The listing builds one solid part. Answer for the finished solid, in the listing's coordinates (mm). Face numbers are marked on the shaded views. Give positions to 0.01 mm unless a question says otherwise; leave off trailing zeros. Loops run counter-clockwise (first coordinate to the right, second up) from the corner with the lowest first, then second, coordinate; pieces in that order, holes last.
Item 1: Section B-B, the plane x = 0 is taken. Give the vertices of the cut face in (y, z).
Item 2: Each of these flat-tipped pins is pushed along its axis until it touches: pin 1 Ø5 at (x, z) = (-7, 7) entering from +Y; pin 2 Ø5 at (y, z) = (4.5, 8) entering from +X; pin 3 Ø4 at (y, z) = (9.5, -2.5) entering from -X; pin 4 Ø5 at (y, z) = (12, -1) entering from -X. Where does it stop, or does it pass through?
Item 3: Section C-C, the plane x = 15 is taken. Give the vertices of the cut face in (y, z).
Item 4: The mould has two halves that part along X. Classify the marked faces 1, 2 and 3: pulls with the +X half, pulls with the -X half, needs draft (parallel to the pull), parting line crosses it, or undercut.
Item 5: Section A-A, the plane y = 1.5 is taken. Give the vertices of the cut face in (x, z).
Item 6: Consider line 1 along Z through (x, y) = (-8, 3); line 2 along X through (y, z) = (10, -3); line 3 along Z through (x, y) = (6, 1.5). Determine where each line is inside the solid, lowest interval first.
from build123d import *

# Parameters (mm, degrees)
BOSS_EXTRUDE1_DEPTH = 15
SKETCH2_R           = 12
CUT_EXTRUDE1_DEPTH  = 28.45639893
CHAMFER1_SIZE       = 1


with BuildPart() as part:
    # Sketch1 → Boss-Extrude1 (new body)
    with BuildSketch(Plane(origin=(0, 0, 0), x_dir=(1, 0, 0), z_dir=(0, 1, 0))):
        Polygon((8.887808978, -14.866299189), (17.318497247, 0.263918764), (8.430688269, 15.130217953), (-8.887808978, 14.866299189), (-17.318497247, -0.263918764), (-8.430688269, -15.130217953), align=None)
    extrude(amount=BOSS_EXTRUDE1_DEPTH)

    # Sketch2 → Cut-Extrude1 (cut, through all)
    with BuildSketch(Plane(origin=(0, 15, 0), x_dir=(1, 0, 0), z_dir=(0, 1, 0))):
        with Locations(Location((0, 0, 0), (0, 0, 270))):
            Circle(SKETCH2_R)
    extrude(amount=-CUT_EXTRUDE1_DEPTH, mode=Mode.SUBTRACT)

    # Chamfer1
    chamfer1_edges = [part.edges().sort_by_distance(p)[0] for p in [
        (0, 0, -12),
    ]]
    chamfer(chamfer1_edges, length=CHAMFER1_SIZE)


solid = part.part
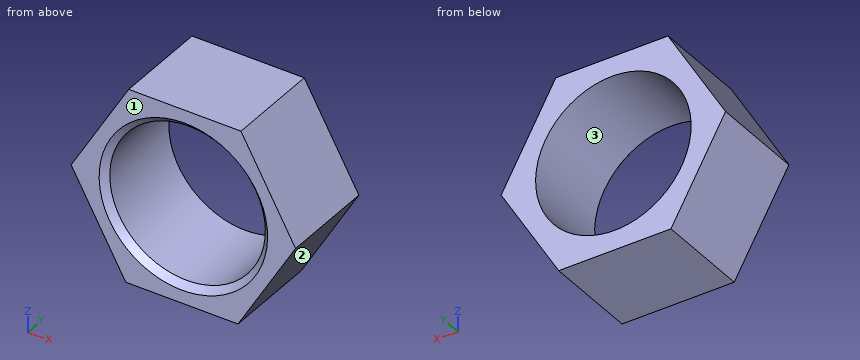
Worked answers:
1. outline: (0, -15) - (15, -15) - (15, -12) - (1, -12) - (0, -13) - close; (0, 13) - (1, 12) - (15, 12) - (15, 15) - (0, 15) - close
2. pin 1: stops at y = 15
2. pin 2: stops at x = 14.11
2. pin 3: stops at x = -16.89
2. pin 4: stops at x = -17.32
3. outline: (0, -4.14) - (15, -4.14) - (15, 3.9) - (0, 3.9) - close
4. face 1: needs draft
4. face 2: pulls with the +X half
4. face 3: undercut
5. outline: (-17.32, 0.26) - (-8.89, -14.87) - (8.43, -15.13) - (17.32, -0.26) - (8.89, 14.87) - (-8.43, 15.13) - close; hole circle Ø24 at (0, 0)
6. line 1: z = -14.88 to -8.94, 8.94 to 15.12
6. line 2: x = -15.5 to -11.62, 11.62 to 15.68
6. line 3: z = -15.09 to -10.39, 10.39 to 14.91
